from build123d import *

# Parameters (mm, degrees)
SKETCH1_W           = 467
SKETCH1_H           = 654
SKETCH1_R           = 10.1
BOSS_EXTRUDE1_DEPTH = 8


with BuildPart() as part:
    # Sketch1 → Boss-Extrude1 (new body)
    with BuildSketch(Plane.XY.offset(8)):
        Rectangle(SKETCH1_W, SKETCH1_H)
        with Locations(Location((144.5, 0, 0), (0, 0, 180))):
            Circle(SKETCH1_R, mode=Mode.SUBTRACT)
    extrude(amount=-BOSS_EXTRUDE1_DEPTH)


solid = part.part
Input: part model. Units: mm. Frame: model coordinates. Give positions to 0.01 mm unless a question says otherwise; leave off trailing zeros. Write each loop counter-clockwise with the first axis right and the second up, starting at its lowest first coordinate (ties: lowest second). Pieces come first, ordered by that corner, then holes.
Q1. Section A-A, the plane x = 144.5. Output: boundary loops of the cut face in (y, z).
Q2. Material intervals for probe 1 along Y at (x, z) = (144.5, 5), sorted ascending.
Q3. First-contact query: P1, Ø8, axis at x = -89, y = -16.5, coming from the -Z side; P2, Ø18, axis at x = 144.5, y = 0, coming from the -Z side. Flat tips, straight axial feed; report the tip coordinate or a pass-through.
Q4. Pull-direction query (X, two-part tool) for faces 1 (the face through (-3, 5, 8)), 2 (the face through (154.59, -0.44, 4.06)); classes: pulls with the +X half, pulls with the -X half, needs draft (parallel to the pull), parting line crosses it, or undercut.
Q5. Section B-B, the plane y = 0. Output: boundary loops of the cut face in (x, z), plus the area to 3 significant figures.
Filled in:
1. outline: (-327, 0) - (-10.1, 0) - (-10.1, 8) - (-327, 8) - close; (10.1, 0) - (327, 0) - (327, 8) - (10.1, 8) - close
2. probe 1: y = -327 to -10.1, 10.1 to 327
3. P1: stops at z = 0
3. P2: passes through
4. face 1: needs draft
4. face 2: undercut
5. outline: (-233.5, 0) - (134.4, 0) - (134.4, 8) - (-233.5, 8) - close; (154.6, 0) - (233.5, 0) - (233.5, 8) - (154.6, 8) - close
5. area: 3,570 mm2
